Solid Edge part; units mm, degrees
sketch "Sketch1" plane through (0, 0, 0) normal (0, -1, 0) x (1, 0, 0)
  arc A0 (7.8125, -39.2296) -> (7.8125, 39.2296) centre (0, 0) cw
  arc A1 (7.8125, 39.2296) -> (242.1875, 39.2296) centre (125, 627.6743) ccw
  arc A2 (242.1875, 39.2296) -> (242.1875, -39.2296) centre (250, 0) cw
  arc A3 (242.1875, -39.2296) -> (7.8125, -39.2296) centre (125, -627.6743) ccw
  dimension "D1" = 39.2296
extrude "Protrusion1" add sketch "Sketch1" against normal blind 15
sketch "Sketch2" plane through (125, 0, 0) normal (0, -1, 0) x (1, 0, 0)
  circle A0 centre (125, 0) radius 22
extrude "Cutout1" cut sketch "Sketch2" against normal through all
hole "Agujero_1" at (250, 0, 32.5) direction (0, 1, 0) diameter 4.917 end up to next
pattern_circular "Pattern1" count 6 over 360 about axis through (250, 0, 0) along (0, 1, 0) of "Agujero_1"
sketch "Sketch3" plane through (125, 0, 0) normal (0, -1, 0) x (1, 0, 0)
  circle A0 centre (-125, 0) radius 3.25
extrude "Cutout2" cut sketch "Sketch3" against normal through all
sketch "Sketch4" plane through (125, 15, 0) normal (0, 1, 0) x (1, 0, 0)
  line L0 (-119, -6) -> (-131, -6)
  line L1 (-131, -6) -> (-131, 6)
  line L2 (-131, 6) -> (-119, 6)
  line L3 (-119, 6) -> (-119, -6)
  dimension "D1" = 131
  dimension "D2" = 119
extrude "VaciadoExtruido_3" cut sketch "Sketch4" against normal blind 12
sketch "Sketch5" plane through (125, 15, 0) normal (0, 1, 0) x (1, 0, 0)
  circle A0 centre (-125, 0) radius 20
extrude "VaciadoExtruido_4" cut sketch "Sketch5" against normal blind 3
hole "Agujero_7" at (-13, 0, 0) direction (0, 1, 0) diameter 4.5 end up to next counterbore diameter 8 counterbore depth 7
pattern_circular "Pattern2" count 6 over 360 about axis through (0, 0, 0) along (0, 1, 0) of "Agujero_7"
hole "Agujero_13" at (48.91, 0, 15) direction (0, 1, 0) diameter 4.917 end up to next
hole "Hole11" at (145.41, 0, 15) direction (0, 1, 0) diameter 4.917 end up to next
hole "Hole12" at (145.41, 0, -15) direction (0, 1, 0) diameter 4.917 end up to next
hole "Hole13" at (48.91, 0, -15) direction (0, 1, 0) diameter 4.917 end up to next
sketch "Sketch6" plane through (125, 0, 0) normal (0, -1, 0) x (1, 0, 0)
  line L0 (7.41, -22) -> (-63.09, -22)
  line L1 (-63.09, -22) -> (-63.09, 22)
  line L2 (-63.09, 22) -> (7.41, 22)
  line L3 (7.41, 22) -> (7.41, -22)
  dimension "D1" = 63.09
  dimension "D2" = 7.41
extrude "Cutout3" cut sketch "Sketch6" against normal through all
fillet "Redondeo_1" radius 5 4 edges at (61.91, 7.5, 22) (132.41, 7.5, 22) (61.91, 7.5, -22) (132.41, 7.5, -22)
properties part number "1976-1300-001" material "Aluminio, 7075-T6"
Geometry: final body of the model. Coordinates: model frame, mm. A direction names the side the tool comes from. Round coordinates to 2 decimals unless told otherwise and drop trailing zeros. Loops run counter-clockwise (first coordinate to the right, second up) from the corner with the lowest first, then second, coordinate; pieces in that order, holes last. Notation, with made-up numbers: M 76.25,50.25 L 135.25,50.25 A30 ccw 135.25,84.25 Z; hole C 33.5,0 d9. An arc over 180 degrees is marked long. Put each result on its own line as item: value. Start each with the question number.
(1) Contact query for flat-ended pins moving along their axis: pin 1 Ø4 at (x, z) = (145.41, -15) entering from +Y; pin 2 Ø1 at (x, y) = (240.5, 6) entering from -Z; pin 3 Ø9.5 at (x, z) = (-0.5, 2) entering from +Y; pin 4 Ø2.5 at (x, z) = (-5, -11.5) entering from -Y. Output: stop coordinate, or through.
(2) Draft query along X for faces 5 (the face through (126.651, 7.395, -27.677)), 6 (the face through (127, 15, 26)). Return one class per face: +X half, -X half, draft (parallel to the pull), parting line (faces both ways), or undercut.
(3) Section query A-A (x = 234). Return loops of the section in (y, z), then the cut area to 3 significant figures.
(4) Set-up query: faces 1 (the face through (-4, 7, -11)), 2 (the face through (123.349, 7.395, 27.677)), 3 (the face through (97, 7, 22)), 4 (the face through (3, 3, -3)). Return all of +Z, -Z, +X, -X, +Y, -Y with unobstructed straight access to the full face (end or side cutting, diameter ignored); none if empty.
(5) Material intervals for line 1 along X through (y, z) = (7.5, -0.5); line 2 along Z through (x, y) = (124.5, 11.25); line 3 along X through (y, z) = (10.25, -19), sorted ascending. Write a range as [from, to].
Findings below:
1. pin 1: passes through
1. pin 2: stops at z = -38.99
1. pin 3: stops at y = 12
1. pin 4: stops at y = 7
2. face 5: undercut
2. face 6: draft
3. outline: M 0,-37.66 L 15,-37.66 L 15,-15.1 L 0,-15.1 Z; M 0,15.1 L 15,15.1 L 15,37.66 L 0,37.66 Z
3. area: 677 mm2
4. face 1: -Y
4. face 2: +Z, +Y, -Y
4. face 3: +Y, -Y
4. face 4: +Y
5. line 1: x = [-40, -15.19], [-10.81, -6], [6, 10.81], [15.19, 61.91], [132.41, 228.01], [271.99, 290]
5. line 2: z = [-27.67, -22], [22, 27.67]
5. line 3: x = [-35.2, 62.33], [131.99, 238.91], [261.09, 285.2]
